For this review, take the finished solid that the model builds, in its own axes (mm). Face numbers are marked on the shaded views. A direction names the side the tool comes from. Give positions to 0.01 mm unless a question says otherwise; leave off trailing zeros. Order: outer loops, then holes, each group sorted by start corner. A loop starts at its lowest first (then second) coordinate and runs counter-clockwise, first axis right, second up. Notation, with made-up numbers: M 16,-25 L 32,-25 A19 ccw 32,9 Z; hole C 82,-16.75 d1. An arc over 180 degrees is marked long. Use CSV: the item, a comma, the result in double quotes. Start each with the question number.
(1) Consider section B-B (x = -13.5). Write out the cut boundary in (y, z).
(2) Tool access review of the marked faces 4 and 5: name each direction out of +Z, -Z, +X, -X, +Y, -Y from which nothing blocks a thin tool from reaching the whole face with its end or side.
(3) Consider section D-D (y = -1). Write out the cut boundary in (x, z), and give its area (3 significant figures).
(4) Wall thickness on L1, parallel to Y at x = 13, z = 6; L2, parallel to X at y = -13, z = 9.25; L3, parallel to X at y = -2.5, z = 3.5: over which ranges is each line inside the solid? List them lowest first. Write a range as from..to.
(5) Consider section C-C (z = 2.25). Write out the cut boundary in (x, y) (3 decimals), and give its area (3 significant figures).
(6) Consider section A-A (x = -10). Write out the cut boundary in (y, z) (3 decimals), and give its area (3 significant figures).
(7) Draft analysis for pull direction Y (two halves, no side actions). For the marked faces 1, 2 and 3, state which applies: pulls with the +Y half, pulls with the -Y half, needs draft (parallel to the pull), parting line crosses it, or undercut.
```python
from build123d import *

# Parameters (mm, degrees)
F0_W           = 34
F0_H           = 38.5
F1_DEPTH       = 10
F3_D           = 4.5
F3_DEPTH       = 10
F3_TIP         = 1.3519363928
F5_D           = 3.5
F5_DEPTH       = 10
F5_CBORE_D     = 8.25
F5_CBORE_DEPTH = 4
F5_TIP         = 1.0515060833


with BuildPart() as f1:
    # F0 (on Top) → F1 (new body)
    with BuildSketch(Plane.XY):
        Rectangle(F0_W, F0_H)
    extrude(amount=F1_DEPTH)

    # F3
    with Locations(Plane(origin=(0, 0, 0), x_dir=(1, 0, 0), z_dir=(0, 0, -1))):
        with Locations((-13, 12.9276185408), (13, 12.9276185408), (-13, -13.0723814592), (13, -13.0723814592)):
            Hole(F3_D / 2, depth=F3_DEPTH)
            with Locations((0, 0, -(F3_DEPTH + F3_TIP / 2))):  # 118° drill point
                Cone(0, F3_D / 2, F3_TIP, mode=Mode.SUBTRACT)

    # F5
    with Locations(Plane(origin=(0, 0, 0), x_dir=(1, 0, 0), z_dir=(0, 0, -1))):
        with Locations((10, 0), (-10, 0)):
            CounterBoreHole(F5_D / 2, F5_CBORE_D / 2, F5_CBORE_DEPTH, depth=F5_DEPTH)
            with Locations((0, 0, -(F5_DEPTH + F5_TIP / 2))):  # 118° drill point
                Cone(0, F5_D / 2, F5_TIP, mode=Mode.SUBTRACT)


solid = f1.part
```
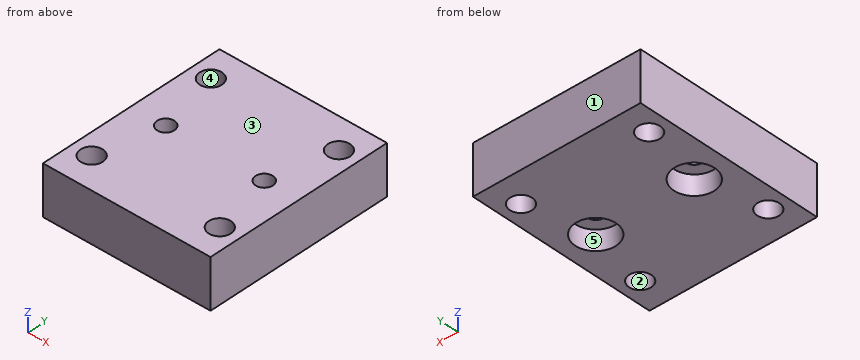
Check result:
1,outline,"M -19.25,0 L -15.12,0 L -15.12,10 L -19.25,10 Z; M -10.73,0 L -2.18,0 L -2.18,4 L 2.18,4 L 2.18,0 L 10.88,0 L 10.88,10 L -10.73,10 Z; M 15.27,0 L 19.25,0 L 19.25,10 L 15.27,10 Z"
2,face 4,"+Z, -Z"
2,face 5,"-Z"
3,outline,"M -17,0 L -14,0 L -14,4 L -11.44,4 L -11.44,10 L -17,10 Z; M -8.56,4 L -6,4 L -6,0 L 6,0 L 6,4 L 8.56,4 L 8.56,10 L -8.56,10 Z; M 11.44,4 L 14,4 L 14,0 L 17,0 L 17,10 L 11.44,10 Z"
3,area,"242 mm^2"
4,L1,"y = -19.25..-15.18, -10.68..10.82, 15.32..19.25"
4,L2,"x = -17..-15.25, -10.75..10.75, 15.25..17"
4,L3,"x = -17..-13.28, -6.72..6.72, 13.28..17"
5,outline,"M -17,-19.25 L 17,-19.25 L 17,19.25 L -17,19.25 Z; hole C -13,-12.928 d4.5; hole C -13,13.072 d4.5; hole C -10,0 d8.25; hole C 10,0 d8.25; hole C 13,-12.928 d4.5; hole C 13,13.072 d4.5"
5,area,"1,140 mm^2"
6,outline,"M -19.25,0 L -4.125,0 L -4.125,4 L -1.75,4 L -1.75,10 L -19.25,10 Z; M 1.75,4 L 4.125,4 L 4.125,0 L 19.25,0 L 19.25,10 L 1.75,10 Z"
6,area,"331 mm^2"
7,face 1,"pulls with the +Y half"
7,face 2,"undercut"
7,face 3,"needs draft"
